For this review, use the dimensioned drawing (mm, ordinates from the lowest corner) and the shaded views. Give positions to 0.01 mm unless a question says otherwise; leave off trailing zeros. Order: outer loops, then holes, each group sorted by start corner. A loop starts at its lowest first (then second) coordinate and runs counter-clockwise, first axis right, second up.
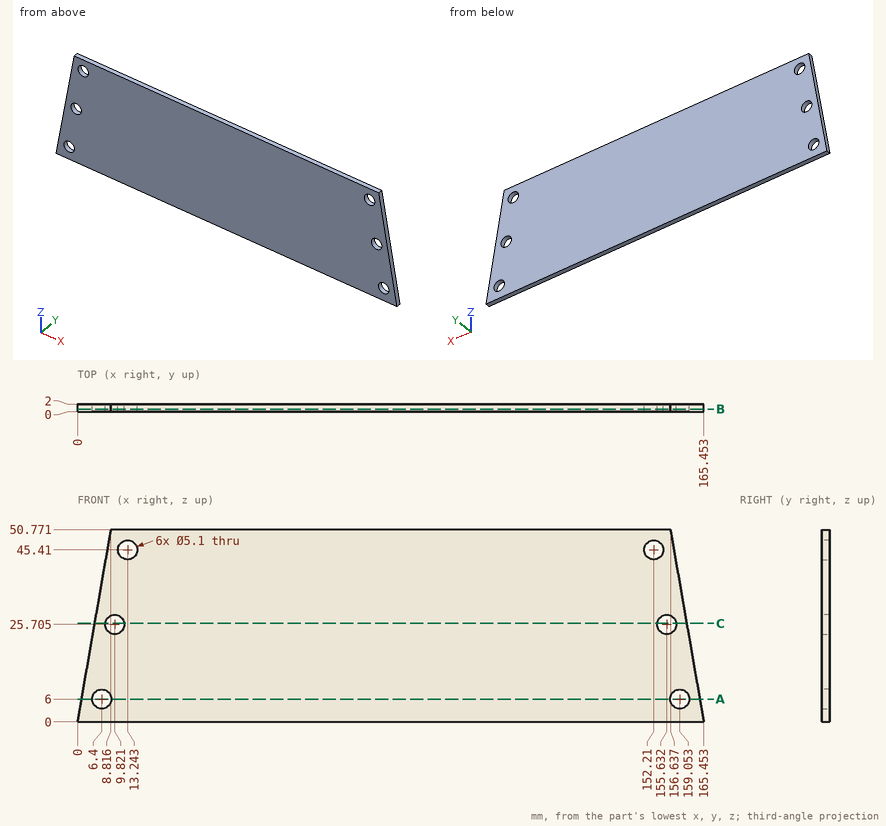
1. For pin 1 (4 mm diameter, centred on x = 13.24, z = 45.41, fed in from -Y) (1 decimal), flat-tipped, find the tip position at first contact; note if it passes through.
Recorded:
pin 1: passes through
2. Take a section at A-A (z = 6). State the section outline as (x, y) points.
Recorded:
outline: (1.04, 0) - (3.85, 0) - (3.85, 2) - (1.04, 2) - close; (8.95, 0) - (156.5, 0) - (156.5, 2) - (8.95, 2) - close; (161.6, 0) - (164.41, 0) - (164.41, 2) - (161.6, 2) - close
3. Take a section at B-B (y = 0.65). State how many separate pieces and enclosed holes the cut face has, then the cut area to 3 significant figures.
Recorded:
separate pieces: 1
enclosed holes: 6
area: 7,830 mm2
4. Take a section at C-C (z = 26). State the section outline as (x, y) points (1 decimal).
Recorded:
outline: (4.5, 0) - (7.3, 0) - (7.3, 2) - (4.5, 2) - close; (12.4, 0) - (153.1, 0) - (153.1, 2) - (12.4, 2) - close; (158.2, 0) - (160.9, 0) - (160.9, 2) - (158.2, 2) - close
5. For line 1 along X through (y, z) = (0.75, 45) (1 decimal); line 2 along X through (y, z) = (0.8, 42); line 3 along X through (y, z) = (1.3, 6), list the stretches that pass through material, from the lowest coordinate up.
Recorded:
line 1: x = 7.8 to 10.7, 15.8 to 149.7, 154.7 to 157.6
line 2: x = 7.29 to 158.16
line 3: x = 1.04 to 3.85, 8.95 to 156.5, 161.6 to 164.41
